Geometry check sheet. Reference: the model listing, model coordinates, mm. Round coordinates to 2 decimals unless told otherwise and drop trailing zeros. Loops run counter-clockwise (first coordinate to the right, second up) from the corner with the lowest first, then second, coordinate; pieces in that order, holes last. Notation, with made-up numbers: (-19, -35.75) - (-4, -35.75) arc R10 cw to (-4, -17.75) - close; hole circle Ø9 at (6.25, 88). An arc over 180 degrees is marked (long way). Answer as CSV lines item,"result". Start each with the question number.
1) Depth check by flat-ended pin: P1, Ø1, axis at x = 1, y = 1.5, coming from the +Z side; P2, Ø1, axis at y = 1, z = -27, coming from the -X side. Enter the tip coordinate at first touch or a pass-through.
2) Thickness scan on line 1 along Z through (x, y) = (5.5, 2.75); line 2 along Z through (x, y) = (1.5, 5); line 3 along Y through (x, z) = (1.5, -5). Record the ranges inside material, lowest first.
3) Cross-section at B-B on x = 1.75. Record the boundary of the cut face in (y, z), and give its area (3 significant figures).
4) Cross-section at A-A on y = 3.75. Record the boundary of the cut face in (x, z), and give its area (3 significant figures).
Autodesk Inventor part; units mm, degrees
ref_plane "YZ Plane" through (0, 0, 0) normal (1, 0, 0) x (0, 1, 0)
ref_plane "XZ Plane" through (0, 0, 0) normal (0, 1, 0) x (-1, 0, 0)
ref_plane "XY Plane" through (0, 0, 0) normal (0, 0, 1) x (1, 0, 0)
sketch "Sketch1" plane through (0, 0, 0) normal (0, 1, 0) x (-1, 0, 0)
  line L0 (0, 0) -> (0, -85)
  line L1 (0, -85) -> (-6.35, -85)
  line L2 (-6.35, -85) -> (-6.35, 0)
  line L3 (-6.35, 0) -> (0, 0)
  dimension "d0" = 85
  dimension "d1" = 6.35
extrude "Extrusion1" add sketch "Sketch1" along normal blind 6.35
sketch "Sketch2" plane through (6.35, 0, 0) normal (1, 0, 0) x (0, 0, -1)
  line L0 (85, 0) -> (0, 0)
  line L1 (0, 0) -> (6.35, 6.35)
  line L2 (85, 6.35) -> (0, 6.35)
  line L3 (0, 0) -> (8.9803, 0) construction
  line L4 (6.35, 6.35) -> (0, 6.35)
  line L5 (0, 6.35) -> (0, 0)
  dimension "d4" = 45
extrude "Extrusion2" cut sketch "Sketch2" against normal blind 10
sketch "Sketch3" plane through (6.35, 0, -85) normal (1, 0, 0) x (0, 0, -1)
  line L0 (0, 0) -> (-6.35, 6.35)
  line L1 (0, 6.35) -> (-78.65, 6.35)
  line L2 (0, 0) -> (8.9803, 0) construction
  line L3 (-6.35, 6.35) -> (0, 6.35)
  line L4 (0, 6.35) -> (0, 0)
  point P0 (-85, 0)
  dimension "d7" = 135
extrude "Extrusion3" cut sketch "Sketch3" against normal blind 10
properties part number "MainAngle"
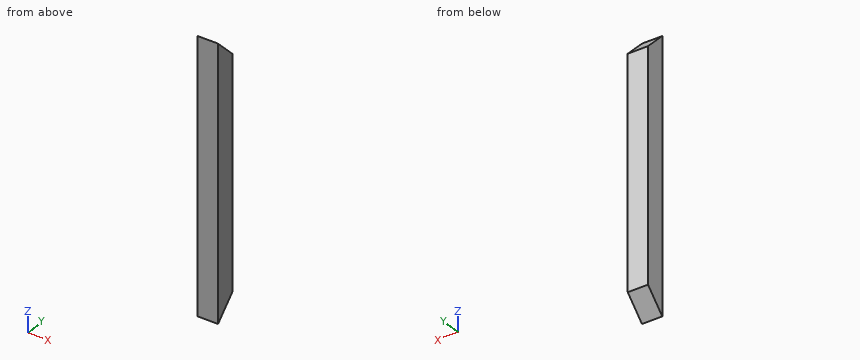
Answer block:
1,P1,"stops at z = -1"
1,P2,"stops at x = 0"
2,line 1,"z = -82.25 to -2.75"
2,line 2,"z = -80 to -5"
2,line 3,"y = 0 to 5"
3,outline,"(0, -85) - (6.35, -78.65) - (6.35, -6.35) - (0, 0) - close"
3,area,"499 mm^2"
4,outline,"(0, -81.25) - (6.35, -81.25) - (6.35, -3.75) - (0, -3.75) - close"
4,area,"492 mm^2"
